```python
from build123d import *


with BuildPart() as part:
    # Sketch1 → Revolve1 (revolve)
    with BuildSketch(Plane(origin=(0, 0, 0), x_dir=(1, 0, 0), z_dir=(0, 1, 0)), mode=Mode.PRIVATE) as revolve1_sk:
        with BuildLine():
            Line((200, 0), (200, 127))
            Line((200, 127), (306, 127))
            Line((306, 127), (585.416444947, 39.563561445))
            ThreePointArc((585.416444947, 39.563561445), (600.17534443, 36.147473842), (615.280908712, 35))
            Line((615.280908712, 35), (645, 35))
            ThreePointArc((645, 35), (675.456211488, 41.825909834), (702.324557443, 57.708788945))
            ThreePointArc((702.324557443, 57.708788945), (705.309695294, 59.409779207), (708.694374787, 60))
            Line((708.694374787, 60), (900, 60))
            Line((900, 60), (900, 0))
            Line((900, 0), (200, 0))
        make_face()
    revolve(revolve1_sk.sketch.rotate(Axis((0, 0, 0), (1, 0, 0)), 180), axis=Axis((0, 0, 0), (1, 0, 0)))


solid = part.part
```
Geometry check sheet. Reference: the model listing, model coordinates, mm. A direction names the side the tool comes from. Coordinates: 2 decimals unless noted, no trailing zeros. Order: outer loops, then holes, each group sorted by start corner. A loop starts at its lowest first (then second) coordinate and runs counter-clockwise, first axis right, second up.
Item 1: Section check D-D (x = 553.5). Enter the section's corners in (y, z), plus the area to 3 significant figures.
Item 2: Tool access check on faces 4 (the conical face through (478.71, -21.914, 69.586)), 5 (the cylindrical face through (253.74, 123.98, -27.53)). Record the directions out of +Z, -Z, +X, -X, +Y, -Y that give a thin tool (end or side, any length) a straight path to the whole face; none if there is none.
Item 3: Depth check by flat-ended pin: pin 1 (6 mm diameter, centred on x = 270.5, y = -56, fed in from -Z); pin 2 (4 mm diameter, centred on x = 642.5, z = -5, fed in from -Y); pin 3 (4 mm diameter, centred on x = 300, y = 25, fed in from +Z). Enter the tip coordinate at first touch or a pass-through.
Item 4: Scan lines: line 1 along X through (y, z) = (-89.5, 85); line 2 along Y through (x, z) = (237, 69); line 3 along Z through (x, y) = (728, -9). Record each from-to range of solid material in increasing order.
Item 5: Mould release check, pull along X, two halves, no side actions. Record for faces 1 (the cylindrical face through (805.69, -50.59, 32.26)), 2 (the flat face through (200, -2, 2)), 3 (the cylindrical face through (630.348, 34.168, -7.587)): released by +X, released by -X, zero draft, split by the parting line, or undercut.
Item 6: Section check A-A (y = 0). Enter the section's corners in (x, z).
Item 7: Section check C-C (x = 658.5). Enter the section's corners in (y, z), plus the area to 3 significant figures.
Check sheet entries:
1. outline: circle Ø99.1 at (0, 0)
1. area: 7,710 mm2
2. face 4: none
2. face 5: +X, -X
3. pin 1: stops at z = -115.41
3. pin 2: stops at y = -34.87
3. pin 3: stops at z = 124.9
4. line 1: x = 200 to 317.4
4. line 2: y = -106.62 to 106.62
4. line 3: z = -59.32 to 59.32
5. face 1: zero draft
5. face 2: released by -X
5. face 3: undercut
6. outline: (200, -127) - (306, -127) - (585.42, -39.56) arc R100 cw to (615.28, -35) - (645, -35) arc R100 cw to (702.32, -57.71) arc R10 ccw to (708.69, -60) - (900, -60) - (900, 60) - (708.69, 60) arc R10 ccw to (702.32, 57.71) arc R100 cw to (645, 35) - (615.28, 35) arc R100 cw to (585.42, 39.56) - (306, 127) - (200, 127) - close
7. outline: circle Ø73.58 at (0, 0)
7. area: 4,250 mm2
